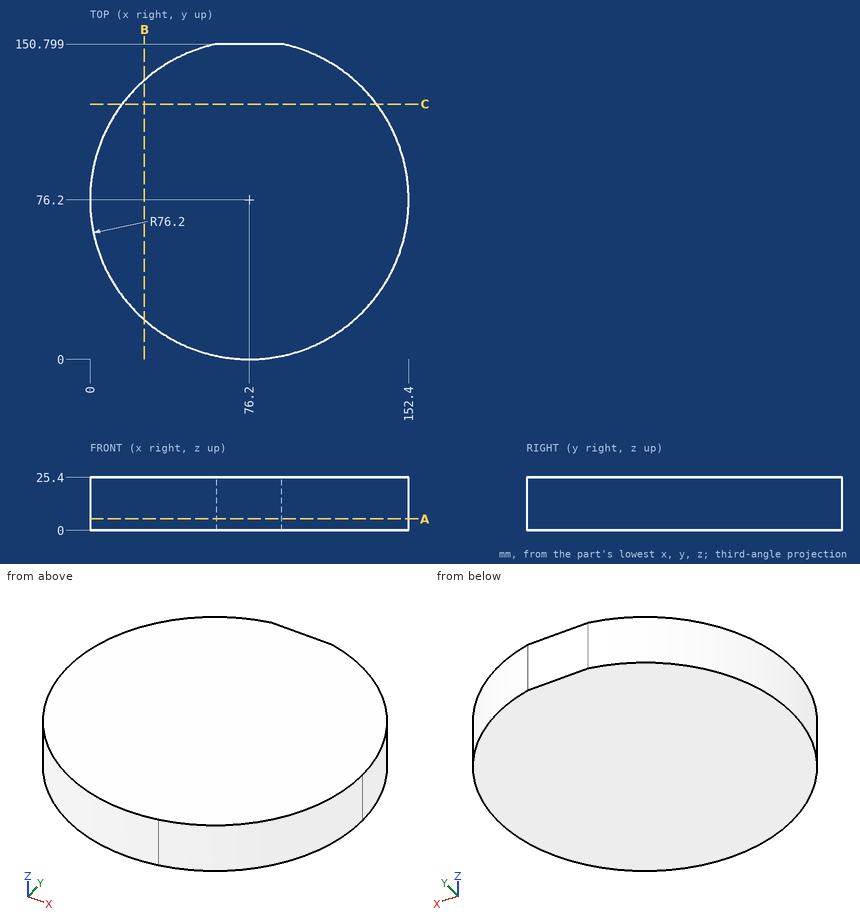
Part print with two shaded views. Sizes in mm from the minimum x, y, z corner. Round coordinates to 2 decimals unless told otherwise and drop trailing zeros. Order: outer loops, then holes, each group sorted by start corner. A loop starts at its lowest first (then second) coordinate and runs counter-clockwise, first axis right, second up. Notation, with made-up numbers: M 35.5,58.25 L 79.5,58.25 A25 cw 79.5,85.25 Z; hole C 1.5,5 d9. An arc over 180 degrees is marked long. Answer in a Markdown table with one row per item. Add a question column.
Q1. Cut at B-B on x = 26. Give the cut face in (y, z).
Q2. Cut at A-A on z = 5.5. Give the cut face in (x, y), and give its area (3 significant figures).
Q3. Cut at C-C on y = 122. Give the cut face in (x, z).
Q4. Pin check, flat tips, straight feed: pin 1 (2 mm diameter, centred on x = 64.5, z = 21, fed in from -Y) (3 decimals); pin 2 (2 mm diameter, centred on y = 28, z = 21.5, fed in from -X); pin 3 (8 mm diameter, centred on y = 124, z = 17.5, fed in from +X). Stop position of each tip, or through.
Q5. Wall check: L1, parallel to X at y = 72.5, z = 9.5; L2, parallel to X at y = 135, z = 21.25; L3, parallel to Y at x = 141.5, z = 12.25. Give the ranges that are in metal, low to high. Write a range as from..to.
Established:
| question | item | result |
|---|---|---|
| 1 | outline | M 18.87,0 L 133.53,0 L 133.53,25.4 L 18.87,25.4 Z |
| 2 | outline | M 60.66,150.8 A76.2 ccw long 91.98,150.75 A76.2 ccw 91.74,150.8 Z |
| 2 | area | 18,200 mm2 |
| 3 | outline | M 15.3,0 L 137.1,0 L 137.1,25.4 L 15.3,25.4 Z |
| 4 | pin 1 | stops at y = 0.755 |
| 4 | pin 2 | stops at x = 16.38 |
| 4 | pin 3 | stops at x = 138.55 |
| 5 | L1 | x = 0.09..152.31 |
| 5 | L2 | x = 27.73..124.67 |
| 5 | L3 | y = 36.93..115.47 |
